Verification items for the finished model (mm, model axes). A direction names the side the tool comes from. Give positions to 0.01 mm unless a question says otherwise; leave off trailing zeros. Loops run counter-clockwise (first coordinate to the right, second up) from the corner with the lowest first, then second, coordinate; pieces in that order, holes last. Notation, with made-up numbers: (65, 73) - (121, 73) arc R33 ccw to (121, 110) - close; hole circle Ø10 at (-18.75, 8.25). An arc over 180 degrees is marked (long way). Use one line per item in the form item = value.
```python
from build123d import *

# Parameters (mm, degrees)
SKETCH_1_W           = 435
SKETCH_1_H           = 200
EXTRUDE_1_DEPTH      = 3
SKETCH_2_R           = 1.6
CUT_EXTRUDE_1_DEPTH  = 157
SKETCH_3_W           = 50
SKETCH_3_H           = 100
CUT_EXTRUDE_2_DEPTH  = 157
SKETCH_5_W           = 20
SKETCH_5_H           = 60
CUT_EXTRUDE_3_DEPTH  = 157
FILLET_1_R           = 5
SKETCH_9_R           = 2.1
CUT_EXTRUDE_6_DEPTH  = 10
SKETCH_10_R          = 1.6
CUT_EXTRUDE_7_DEPTH  = 10
SKETCH_8_R           = 1.75
CUT_EXTRUDE_8_DEPTH  = 10
SKETCH_13_W          = 53.114182181
SKETCH_13_H          = 240.503799042
CUT_EXTRUDE_11_DEPTH = 10
SKETCH_14_W          = 70
SKETCH_14_H          = 75
CUT_EXTRUDE_12_DEPTH = 64.5
FILLET_4_R           = 10
CUT_EXTRUDE_13_DEPTH = 10
EXTRUDE_3_DEPTH      = 3


with BuildPart() as part:
    # 草图1 → 凸台-拉伸1 (new body)
    with BuildSketch(Plane(origin=(0, 0, 0), x_dir=(1, 0, 0), z_dir=(0, 1, 0))):
        Rectangle(SKETCH_1_W, SKETCH_1_H)
    extrude(amount=EXTRUDE_1_DEPTH)

    # 草图2 → 切除-拉伸1 (cut)
    with BuildSketch(Plane(origin=(0, 3, 0), x_dir=(1, 0, 0), z_dir=(0, 1, 0))):
        with Locations(Location((138.5, 16.75, 0), (0, 0, 270))):
            Circle(SKETCH_2_R)
        with Locations(Location((138.5, -56.75, 0), (0, 0, 270))):
            Circle(SKETCH_2_R)
        with Locations(Location((81.5, -56.75, 0), (0, 0, 270))):
            Circle(SKETCH_2_R)
        with Locations(Location((81.5, 16.75, 0), (0, 0, 270))):
            Circle(SKETCH_2_R)
        with Locations(Location((-81.5, 16.75, 0), (0, 0, 270))):
            Circle(SKETCH_2_R)
        with Locations(Location((-81.5, -56.75, 0), (0, 0, 270))):
            Circle(SKETCH_2_R)
        with Locations(Location((-138.5, -56.75, 0), (0, 0, 270))):
            Circle(SKETCH_2_R)
        with Locations(Location((-138.5, 16.75, 0), (0, 0, 270))):
            Circle(SKETCH_2_R)
    extrude(amount=-CUT_EXTRUDE_1_DEPTH, mode=Mode.SUBTRACT)

    # 草图3 → 切除-拉伸2 (cut)
    with BuildSketch(Plane(origin=(0, 3, 0), x_dir=(1, 0, 0), z_dir=(0, 1, 0))):
        with Locations((-110, -20)):
            Rectangle(SKETCH_3_W, SKETCH_3_H)
        with Locations((110, -20)):
            Rectangle(SKETCH_3_W, SKETCH_3_H)
    extrude(amount=-CUT_EXTRUDE_2_DEPTH, mode=Mode.SUBTRACT)

    # 草图5 → 切除-拉伸3 (cut)
    with BuildSketch(Plane(origin=(0, 3, 0), x_dir=(1, 0, 0), z_dir=(0, 1, 0))):
        with Locations((-145, -20)):
            Rectangle(SKETCH_5_W, SKETCH_5_H)
        with Locations((145, -20)):
            Rectangle(SKETCH_5_W, SKETCH_5_H)
    extrude(amount=-CUT_EXTRUDE_3_DEPTH, mode=Mode.SUBTRACT)

    # 圆角1
    fillet_1_edges = [part.edges().sort_by_distance(p)[0] for p in [
        (135, 1.5, -10),
        (135, 1.5, 50),
        (155, 1.5, -10),
        (155, 1.5, 50),
        (-85, 1.5, -30),
        (-85, 1.5, 70),
        (-135, 1.5, 70),
        (-135, 1.5, -30),
        (135, 1.5, -30),
        (135, 1.5, 70),
        (85, 1.5, 70),
        (85, 1.5, -30),
        (-135, 1.5, -10),
        (-135, 1.5, 50),
        (-155, 1.5, 50),
        (-155, 1.5, -10),
    ]]
    fillet(fillet_1_edges, radius=FILLET_1_R)

    # 草图9 → 切除-拉伸6 (cut)
    with BuildSketch(Plane(origin=(0, 3, 0), x_dir=(1, 0, 0), z_dir=(0, 1, 0))):
        with Locations(Location((-137.5, -85, 0), (0, 0, 270))):
            Circle(SKETCH_9_R)
        with Locations(Location((-57.5, -85, 0), (0, 0, 270))):
            Circle(SKETCH_9_R)
        with Locations(Location((57.5, -85, 0), (0, 0, 270))):
            Circle(SKETCH_9_R)
        with Locations(Location((137.5, -85, 0), (0, 0, 270))):
            Circle(SKETCH_9_R)
        with Locations(Location((137.5, 85, 0), (0, 0, 270))):
            Circle(SKETCH_9_R)
        with Locations(Location((57.5, 85, 0), (0, 0, 270))):
            Circle(SKETCH_9_R)
        with Locations(Location((-57.5, 85, 0), (0, 0, 270))):
            Circle(SKETCH_9_R)
        with Locations(Location((-137.5, 85, 0), (0, 0, 270))):
            Circle(SKETCH_9_R)
    extrude(amount=-CUT_EXTRUDE_6_DEPTH, mode=Mode.SUBTRACT)

    # 草图10 → 切除-拉伸7 (cut)
    with BuildSketch(Plane(origin=(0, 3, 0), x_dir=(1, 0, 0), z_dir=(0, 1, 0))):
        with Locations(Location((-25, -15, 0), (0, 0, 270))):
            Circle(SKETCH_10_R)
        with Locations(Location((25, -15, 0), (0, 0, 270))):
            Circle(SKETCH_10_R)
        with Locations(Location((25, -65, 0), (0, 0, 270))):
            Circle(SKETCH_10_R)
        with Locations(Location((-25, -65, 0), (0, 0, 270))):
            Circle(SKETCH_10_R)
    extrude(amount=-CUT_EXTRUDE_7_DEPTH, mode=Mode.SUBTRACT)

    # 草图8 → 切除-拉伸8 (cut)
    with BuildSketch(Plane(origin=(0, 3, 0), x_dir=(1, 0, 0), z_dir=(0, 1, 0))):
        with Locations(Location((-35.85, 49.25, 0), (0, 0, 270))):
            Circle(SKETCH_8_R)
        with Locations(Location((35.85, 49.25, 0), (0, 0, 270))):
            Circle(SKETCH_8_R)
        with Locations(Location((-35.85, 20.75, 0), (0, 0, 270))):
            Circle(SKETCH_8_R)
        with Locations(Location((35.85, 20.75, 0), (0, 0, 270))):
            Circle(SKETCH_8_R)
    extrude(amount=-CUT_EXTRUDE_8_DEPTH, mode=Mode.SUBTRACT)

    # 草图13 → 切除-拉伸11 (cut)
    with BuildSketch(Plane(origin=(0, 3, 0), x_dir=(1, 0, 0), z_dir=(0, 1, 0))):
        with BuildLine():
            Line((-46.500708687, -60), (-46.500708687, 60))
            ThreePointArc((-46.500708687, 60), (-48.258068, 64.242640687), (-52.500708687, 66))
            Line((-52.500708687, 66), (-142.500708687, 66))
            ThreePointArc((-142.500708687, 66), (-148.500708687, 60), (-142.500708687, 54))
            Line((-142.500708687, 54), (-58.500708687, 54))
            Line((-58.500708687, 54), (-58.500708687, -60))
            ThreePointArc((-58.500708687, -60), (-52.500708687, -66), (-46.500708687, -60))
        make_face()
        with BuildLine():
            ThreePointArc((52.500708687, 66), (48.258068, 64.242640687), (46.500708687, 60))
            Line((46.500708687, 60), (46.500708687, -60))
            ThreePointArc((46.500708687, -60), (52.500708687, -66), (58.500708687, -60))
            Line((58.500708687, -60), (58.500708687, 54))
            Line((58.500708687, 54), (142.500708687, 54))
            ThreePointArc((142.500708687, 54), (148.500708687, 60), (142.500708687, 66))
            Line((142.500708687, 66), (52.500708687, 66))
        make_face()
        with BuildLine():
            Line((20, 8), (-20, 8))
            ThreePointArc((-20, 8), (-28, 0), (-20, -8))
            Line((-20, -8), (20, -8))
            ThreePointArc((20, -8), (28, 0), (20, 8))
        make_face()
        with Locations((-196.557091091, 5.612879566)):
            Rectangle(SKETCH_13_W, SKETCH_13_H)
        with Locations((196.557091091, 5.612879566)):
            Rectangle(SKETCH_13_W, SKETCH_13_H)
    extrude(amount=-CUT_EXTRUDE_11_DEPTH, mode=Mode.SUBTRACT)

    # 草图14 → 切除-拉伸12 (cut)
    with BuildSketch(Plane(origin=(0, 3, 0), x_dir=(1, 0, 0), z_dir=(0, 1, 0))):
        with Locations((0, 100)):
            Rectangle(SKETCH_14_W, SKETCH_14_H)
    extrude(amount=-CUT_EXTRUDE_12_DEPTH, mode=Mode.SUBTRACT)

    # 圆角4
    fillet_4_edges = [part.edges().sort_by_distance(p)[0] for p in [
        (170, 1.5, 100),
        (-170, 1.5, 100),
        (-170, 1.5, -100),
        (170, 1.5, -100),
        (-35, 1.5, -100),
        (35, 1.5, -100),
        (35, 1.5, -62.5),
        (-35, 1.5, -62.5),
    ]]
    fillet(fillet_4_edges, radius=FILLET_4_R)

    # 草图15 → 切除-拉伸13 (cut)
    with BuildSketch(Plane(origin=(0, 3, 0), x_dir=(1, 0, 0), z_dir=(0, 1, 0))):
        with BuildLine():
            Line((-6.953821544, -32.381919427), (-10.478523956, -22.69787914))
            ThreePointArc((-10.478523956, -22.69787914), (-12.675221062, -19.835087734), (-16.11667968, -18.75))
            Line((-16.11667968, -18.75), (-19.915434451, -18.75))
            ThreePointArc((-19.915434451, -18.75), (-22.743861576, -19.921572875), (-23.915434451, -22.75))
            Line((-23.915434451, -22.75), (-23.915434451, -31.75))
            ThreePointArc((-23.915434451, -31.75), (-22.158075138, -35.992640687), (-17.915434451, -37.75))
            Line((-17.915434451, -37.75), (-10.712592027, -37.75))
            ThreePointArc((-10.712592027, -37.75), (-7.43598385, -36.044305745), (-6.953821544, -32.381919427))
        make_face()
        with BuildLine():
            Line((3.71555598, -18.75), (-3.71555598, -18.75))
            ThreePointArc((-3.71555598, -18.75), (-6.173012113, -20.029270691), (-6.534633842, -22.77606043))
            Line((-6.534633842, -22.77606043), (-1.563535714, -36.434040287))
            ThreePointArc((-1.563535714, -36.434040287), (-0.957470976, -37.29228885), (0, -37.724902295))
            ThreePointArc((0, -37.724902295), (0.957470976, -37.29228885), (1.563535714, -36.434040287))
            Line((1.563535714, -36.434040287), (6.534633842, -22.77606043))
            ThreePointArc((6.534633842, -22.77606043), (6.173012113, -20.029270691), (3.71555598, -18.75))
        make_face()
        with BuildLine():
            Line((19.915434451, -18.75), (16.11667968, -18.75))
            ThreePointArc((16.11667968, -18.75), (12.675221062, -19.835087734), (10.478523956, -22.69787914))
            Line((10.478523956, -22.69787914), (6.953821544, -32.381919427))
            ThreePointArc((6.953821544, -32.381919427), (7.43598385, -36.044305745), (10.712592027, -37.75))
            Line((10.712592027, -37.75), (17.915434451, -37.75))
            ThreePointArc((17.915434451, -37.75), (22.158075138, -35.992640687), (23.915434451, -31.75))
            Line((23.915434451, -31.75), (23.915434451, -22.75))
            ThreePointArc((23.915434451, -22.75), (22.743861576, -19.921572875), (19.915434451, -18.75))
        make_face()
        with BuildLine():
            Line((6.953821544, -47.618080573), (10.478523956, -57.30212086))
            ThreePointArc((10.478523956, -57.30212086), (12.675221062, -60.164912266), (16.11667968, -61.25))
            Line((16.11667968, -61.25), (19.915434451, -61.25))
            ThreePointArc((19.915434451, -61.25), (22.743861576, -60.078427125), (23.915434451, -57.25))
            Line((23.915434451, -57.25), (23.915434451, -48.25))
            ThreePointArc((23.915434451, -48.25), (22.158075138, -44.007359313), (17.915434451, -42.25))
            Line((17.915434451, -42.25), (10.712592027, -42.25))
            ThreePointArc((10.712592027, -42.25), (7.43598385, -43.955694255), (6.953821544, -47.618080573))
        make_face()
        with BuildLine():
            Line((-3.71555598, -61.25), (3.71555598, -61.25))
            ThreePointArc((3.71555598, -61.25), (6.173012113, -59.970729309), (6.534633842, -57.22393957))
            Line((6.534633842, -57.22393957), (1.563535714, -43.565959713))
            ThreePointArc((1.563535714, -43.565959713), (0.957470976, -42.70771115), (0, -42.275097705))
            ThreePointArc((0, -42.275097705), (-0.957470976, -42.70771115), (-1.563535714, -43.565959713))
            Line((-1.563535714, -43.565959713), (-6.534633842, -57.22393957))
            ThreePointArc((-6.534633842, -57.22393957), (-6.173012113, -59.970729309), (-3.71555598, -61.25))
        make_face()
        with BuildLine():
            Line((-10.712592027, -42.25), (-17.915434451, -42.25))
            ThreePointArc((-17.915434451, -42.25), (-22.158075138, -44.007359313), (-23.915434451, -48.25))
            Line((-23.915434451, -48.25), (-23.915434451, -57.25))
            ThreePointArc((-23.915434451, -57.25), (-22.743861576, -60.078427125), (-19.915434451, -61.25))
            Line((-19.915434451, -61.25), (-16.11667968, -61.25))
            ThreePointArc((-16.11667968, -61.25), (-12.675221062, -60.164912266), (-10.478523956, -57.30212086))
            Line((-10.478523956, -57.30212086), (-6.953821544, -47.618080573))
            ThreePointArc((-6.953821544, -47.618080573), (-7.43598385, -43.955694255), (-10.712592027, -42.25))
        make_face()
    extrude(amount=-CUT_EXTRUDE_13_DEPTH, mode=Mode.SUBTRACT)

    # 草图16 → 凸台-拉伸3 (add)
    with BuildSketch(Plane(origin=(0, 3, 0), x_dir=(1, 0, 0), z_dir=(0, 1, 0))):
        with BuildLine():
            Line((-46.500708687, 60), (-58.500708687, 48))
            Line((-58.500708687, 48), (-58.500708687, 54))
            Line((-58.500708687, 54), (-64.500708687, 54))
            Line((-64.500708687, 54), (-52.500708687, 66))
            ThreePointArc((-52.500708687, 66), (-48.258068, 64.242640687), (-46.500708687, 60))
        make_face()
        with BuildLine():
            ThreePointArc((46.500708687, 60), (48.258068, 64.242640687), (52.500708687, 66))
            Line((52.500708687, 66), (64.500708687, 54))
            Line((64.500708687, 54), (58.500708687, 54))
            Line((58.500708687, 54), (58.500708687, 48))
            Line((58.500708687, 48), (46.500708687, 60))
        make_face()
    extrude(amount=-EXTRUDE_3_DEPTH)


solid = part.part
```
1. Tool access check on faces 4 (the cylindrical face through (-28, 2, 0)), 5 (the cylindrical face through (-38.01, 1.48, -97.15)), 6 (the flat face through (2, 3, -24)). Record the directions out of +Z, -Z, +X, -X, +Y, -Y that give a thin tool (end or side, any length) a straight path to the whole face; none if there is none.
Result set:
face_4 = +Y, -Y
face_5 = -Z, +Y, -Y
face_6 = +Z, -Z, +X, -X, +Y
2. Section check A-A, the plane x = 70. Record the cut outline in (y, z).
Result set:
outline = (0, -100) - (3, -100) - (3, -66) - (0, -66) - close; (0, -54) - (3, -54) - (3, 100) - (0, 100) - close
3. Draft check along Z on faces 1 (the cylindrical face through (28, 2, 0)), 2 (the flat face through (2, 0, -24)), 3 (the cylindrical face through (-32.15, 1.48, -65.51)). Enter one of: released by +Z, released by -Z, zero draft, split by the parting line, or undercut.
Result set:
face_1 = undercut
face_2 = zero draft
face_3 = released by -Z
4. Depth check by flat-ended pin: pin 1 Ø4 at (x, z) = (-57.5, 85) entering from -Y. Enter the tip coordinate at first touch or a pass-through.
Result set:
pin_1 = through
5. Section check B-B, the plane y = 1.75. State how many separate pieces and enclosed holes the cut face has, then the cut area to 3 significant figures.
Result set:
separate_pieces = 1
enclosed_holes = 37
area = 45,500 mm²
6. Scan lines: probe 1 along X at (y, z) = (1.9, 7); probe 2 along X at (y, z) = (1, -85); probe 3 along X at (y, z) = (2.15, 85). Record each from-to range of solid material in increasing order.
Result set:
probe_1 = -170 to -155, -85 to -58.5, -46.5 to -23.87, 23.87 to 46.5, 58.5 to 85, 155 to 170
probe_2 = -170 to -139.6, -135.4 to -59.6, -55.4 to -35, 35 to 55.4, 59.6 to 135.4, 139.6 to 170
probe_3 = -170 to -139.6, -135.4 to -59.6, -55.4 to 55.4, 59.6 to 135.4, 139.6 to 170
